Source: CAD feature listing. Evaluate the final solid. Frame: model axes, mm. Face numbers are marked on the shaded views. A direction names the side the tool comes from. Give positions to 0.01 mm unless a question says otherwise; leave off trailing zeros. Order: outer loops, then holes, each group sorted by start corner. A loop starts at its lowest first (then second) coordinate and runs counter-clockwise, first axis right, second up.
1) Material intervals for line 1 (X direction, y = 10, z = 0); line 2 (X direction, y = 1.6, z = 0); line 3 (Y direction, x = -12, z = -4.5), sorted ascending.
2) First-contact query: P1, Ø5, axis at y = 2, z = -8.5, coming from the +X side; P2, Ø5, axis at x = 1.5, z = -24.5, coming from the -Y side; P3, Ø4, axis at y = 4, z = 3.5, coming from the +X side; P4, Ø2, axis at x = -16.5, y = 8, coming from the -Z side. Flat tips, straight axial feed; report the tip coordinate or a pass-through.
3) Draft query along X for the marked faces 6, 7 and 8. Return one class per face: released by +X, released by -X, zero draft, split by the parting line, or undercut.
4) Access query for the marked faces 1, 2, 3, 4 and 5. Directions: +Z, -Z, +X, -X, +Y, -Y. A direction counts if a zero-diameter tool reaches every point of the face in a straight line with its end or side. Return the directions, or none.
5) Section B-B, the plane x = 0. Give the number of separate pieces and of enclosed holes in the cut face, plus the area to 3 significant figures.
6) Section C-C, the plane z = -24.15. Return loops of the section in (x, y).
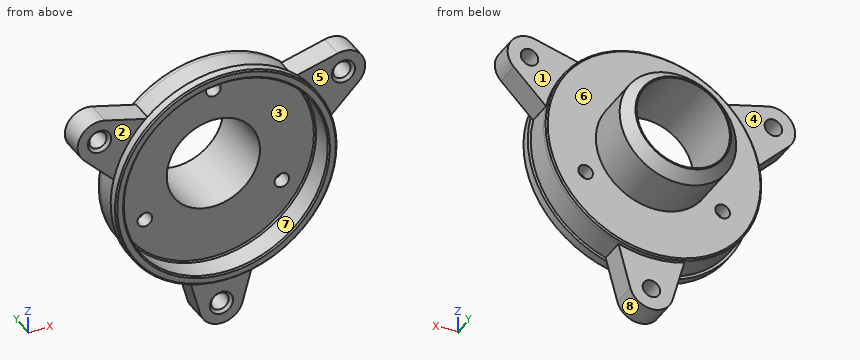
```python
from build123d import *

# Parameters (mm, degrees)
SKETCH1_R               = 1.5
BOSS_EXTRUDE1_DEPTH     = 4.3
SKETCH3_R               = 18.5
BOSS_EXTRUDE2_DEPTH     = 0.9
CUT_EXTRUDE1_DEPTH      = 38.486507256
CUT_EXTRUDE1_DEPTH_BACK = 38.486507256
SKETCH2_R               = 1.25
SKETCH4_R               = 10
BOSS_EXTRUDE3_DEPTH     = 9.75
SKETCH5_R               = 8
CUT_EXTRUDE2_DEPTH      = 41.127929504
SKETCH6_R               = 19
BOSS_EXTRUDE4_DEPTH     = 1.7
SKETCH7_R               = 17.5
CUT_EXTRUDE3_DEPTH      = 4.4
CHAMFER1_SIZE           = 1.8
CHAMFER2_SIZE           = 0.25
CHAMFER3_SIZE           = 0.5


with BuildPart() as part:
    # Sketch1 → Boss-Extrude1 (new body)
    with BuildSketch(Plane(origin=(0, 0, 0), x_dir=(1, 0, 0), z_dir=(0, 1, 0))):
        with BuildLine():
            Line((-3.620168852, 25.128201147), (-5.65, 17.616114782))
            ThreePointArc((-5.65, 17.616114782), (-16.02146997, 9.25), (-18.081002917, -3.915013859))
            Line((-18.081002917, -3.915013859), (-23.57174497, -9.428942382))
            ThreePointArc((-23.57174497, -9.428942382), (-24.162108766, -13.95), (-19.951576119, -15.699258765))
            Line((-19.951576119, -15.699258765), (-12.431002917, -13.701100922))
            ThreePointArc((-12.431002917, -13.701100922), (0, -18.5), (12.431002917, -13.701100922))
            Line((12.431002917, -13.701100922), (19.951576119, -15.699258765))
            ThreePointArc((19.951576119, -15.699258765), (24.162108766, -13.95), (23.57174497, -9.428942382))
            Line((23.57174497, -9.428942382), (18.081002917, -3.915013859))
            ThreePointArc((18.081002917, -3.915013859), (16.02146997, 9.25), (5.65, 17.616114782))
            Line((5.65, 17.616114782), (3.620168852, 25.128201147))
            ThreePointArc((3.620168852, 25.128201147), (0, 27.9), (-3.620168852, 25.128201147))
        make_face()
        with Locations(Location((0, 24.15, 0), (0, 0, 90))):
            Circle(SKETCH1_R, mode=Mode.SUBTRACT)
        with Locations(Location((20.914513501, -12.075, 0), (0, 0, 90))):
            Circle(SKETCH1_R, mode=Mode.SUBTRACT)
        with Locations(Location((-20.914513501, -12.075, 0), (0, 0, 90))):
            Circle(SKETCH1_R, mode=Mode.SUBTRACT)
    extrude(amount=BOSS_EXTRUDE1_DEPTH)

    # Sketch3 → Boss-Extrude2 (add)
    with BuildSketch(Plane(origin=(0, 4.3, 0), x_dir=(1, 0, 0), z_dir=(0, 1, 0))):
        with Locations(Location((0, 0, 0), (0, 0, 72.217444278))):
            Circle(SKETCH3_R)
    extrude(amount=BOSS_EXTRUDE2_DEPTH)

    # Sketch2 → Cut-Extrude1 (cut, two sides: drawn at the far end of the back side and taken through both)
    with BuildSketch(Plane(origin=(0, 4.3, 0), x_dir=(1, 0, 0), z_dir=(0, 1, 0)).offset(-CUT_EXTRUDE1_DEPTH_BACK)):
        with Locations(Location((-11.75, 6.783865663, 0), (0, 0, 270))):
            Circle(SKETCH2_R)
        with Locations(Location((11.75, 6.783865663, 0), (0, 0, 270))):
            Circle(SKETCH2_R)
        with Locations(Location((0, -13.567731326, 0), (0, 0, 270))):
            Circle(SKETCH2_R)
    extrude(amount=CUT_EXTRUDE1_DEPTH + CUT_EXTRUDE1_DEPTH_BACK, mode=Mode.SUBTRACT)

    # Sketch4 → Boss-Extrude3 (add)
    with BuildSketch(Plane(origin=(0, 5.2, 0), x_dir=(1, 0, 0), z_dir=(0, 1, 0))):
        with Locations(Location((0, 0, 0), (0, 0, 270))):
            Circle(SKETCH4_R)
    extrude(amount=BOSS_EXTRUDE3_DEPTH)

    # Sketch5 → Cut-Extrude2 (cut, through all)
    with BuildSketch(Plane(origin=(0, 14.95, 0), x_dir=(1, 0, 0), z_dir=(0, 1, 0))):
        with Locations(Location((0, 0, 0), (0, 0, 270))):
            Circle(SKETCH5_R)
    extrude(amount=-CUT_EXTRUDE2_DEPTH, mode=Mode.SUBTRACT)

    # Sketch6 → Boss-Extrude4 (add)
    with BuildSketch(Plane.XZ):
        with Locations(Location((0, 0, 0), (0, 0, 46.812273556))):
            Circle(SKETCH6_R)
    extrude(amount=BOSS_EXTRUDE4_DEPTH)

    # Sketch7 → Cut-Extrude3 (cut)
    with BuildSketch(Plane(origin=(0, -1.7, 0), x_dir=(-1, 0, 0), z_dir=(0, -1, 0))):
        with Locations(Location((0, 0, 0), (0, 0, 90))):
            Circle(SKETCH7_R)
    extrude(amount=-CUT_EXTRUDE3_DEPTH, mode=Mode.SUBTRACT)

    # Chamfer1
    chamfer1_edges = [part.edges().sort_by_distance(p)[0] for p in [
        (0, 14.95, -10),
    ]]
    chamfer(chamfer1_edges, length=CHAMFER1_SIZE)

    # Chamfer2
    chamfer2_edges = [part.edges().sort_by_distance(p)[0] for p in [
        (0, -1.7, 17.5),
        (0, 2.7, 17.5),
        (-5.65, 5.2, 17.616114782),
        (-13.003427764, -1.7, -13.853189755),
    ]]
    chamfer(chamfer2_edges, length=CHAMFER2_SIZE)

    # Chamfer3
    chamfer3_edges = [part.edges().sort_by_distance(p)[0] for p in [
        (0, 0, -22.65),
        (20.914513501, 0, 13.575),
        (-20.914513501, 0, 13.575),
    ]]
    chamfer(chamfer3_edges, length=CHAMFER3_SIZE)


solid = part.part
```
From the geometry:
1. line 1: x = -10 to -8, 8 to 10
1. line 2: x = -18.5 to -17.5, 17.5 to 18.5
1. line 3: y = 2.7 to 5.2
2. P1: stops at x = 17.66
2. P2: stops at y = 0
2. P3: stops at x = 19.66
2. P4: passes through
3. face 6: zero draft
3. face 7: undercut
3. face 8: split by the parting line
4. face 1: +Z, +X, +Y
4. face 2: +Z, -X, -Y
4. face 3: -Y
4. face 4: +Z, -X, +Y
4. face 5: +Z, +X, -Y
5. separate pieces: 4
5. enclosed holes: 0
5. area: 120 mm2
6. outline: (-3.88, 0) - (-2, 0) - (-1.5, 0.5) - (-1.5, 4.3) - (-3.88, 4.3) - close; (1.5, 0.5) - (2, 0) - (3.88, 0) - (3.88, 4.3) - (1.5, 4.3) - close
